Autodesk Inventor part; units mm, degrees
ref_plane "YZ Plane" through (0, 0, 0) normal (1, 0, 0) x (0, 1, 0)
ref_plane "XZ Plane" through (0, 0, 0) normal (0, 1, 0) x (-1, 0, 0)
ref_plane "XY Plane" through (0, 0, 0) normal (0, 0, 1) x (1, 0, 0)
sketch "Sketch1" plane through (0, 0, 0) normal (0, 0, 1) x (1, 0, 0)
  circle A0 centre (0, 0) radius 3.5
  dimension "d0" = 7
extrude "Extrusion1" add sketch "Sketch1" along normal blind 70
sketch "Sketch2" plane through (0, 0, 0) normal (0, 0, -1) x (-1, 0, 0)
  circle A0 centre (0, 0) radius 3.5
  line L0 (-2, 2.8723) -> (-2, 4.8723)
  line L1 (-2, 4.8723) -> (2, 4.8723)
  line L2 (2, 4.8723) -> (2, 2.8723)
  arc A1 (2, 2.8723) -> (-2, 2.8723) centre (0, 0) ccw
  point P0 (0, 4.8723)
  dimension "d3" = 4
  dimension "d4" = 2
extrude "Extrusion2" add sketch "Sketch2" against normal blind 20 contours A0 L0 L1 L2
properties part number "shaft1"
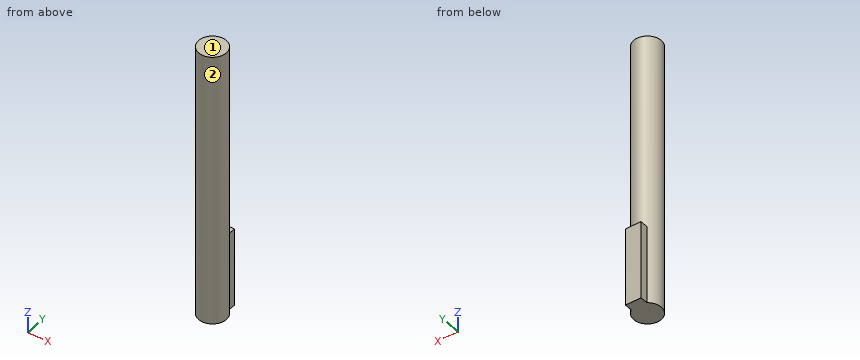
Build history of the part. All positions in model axes, mm. Face numbers are marked on the shaded views. A direction names the side the tool comes from. Round coordinates to 2 decimals unless told otherwise and drop trailing zeros. Loops run counter-clockwise (first coordinate to the right, second up) from the corner with the lowest first, then second, coordinate; pieces in that order, holes last.
Item 1: Saw through at B-B (z = 61.5). List the corners of the cut face in (x, y).
Item 2: Which spindle directions (+Z, -Z, +X, -X, +Y, -Y) get a long thin tool onto all of the face, cutting with end or side? Do the marked faces 1 and 2. Say none if no direction does.
Item 3: Pin check, flat tips, straight feed: P1, Ø1.5, axis at y = 1, z = 7.5, coming from the +X side; P2, Ø1.5, axis at x = -2, z = 46, coming from the +Y side; P3, Ø1, axis at y = 4, z = 13, coming from the -X side. Stop position of each tip, or through.
Item 4: Drill centre lines: line 1 along Y through (x, z) = (0, 63.5); line 2 along Z through (x, y) = (-0.5, 4.5); line 3 along X through (y, z) = (-1.5, 31). Where is each one in solid material? Low to high.
Item 5: Saw through at A-A (x = 0). List the corners of the cut face in (y, z), then the cut area to 3 significant figures.
Item 6: Saw through at C-C (z = 12). List the corners of the cut face in (x, y).
Worked answers:
1. outline: circle Ø7 at (0, 0)
2. face 1: +Z, +X, -X, +Y, -Y
2. face 2: +Z
3. P1: stops at x = 3.49
3. P2: stops at y = 3.27
3. P3: stops at x = -2
4. line 1: y = -3.5 to 3.5
4. line 2: z = 0 to 20
4. line 3: x = -3.16 to 3.16
5. outline: (-3.5, 0) - (4.87, 0) - (4.87, 20) - (3.5, 20) - (3.5, 70) - (-3.5, 70) - close
5. area: 517 mm2
6. outline: (-2, 2.87) arc R3.5 ccw (long way) to (2, 2.87) - (2, 4.87) - (-2, 4.87) - close
